Design review of the part built by this model. Coordinates are the model's own, in mm. A direction names the side the tool comes from. Give positions to 0.01 mm unless a question says otherwise; leave off trailing zeros. Write each loop counter-clockwise with the first axis right and the second up, starting at its lowest first coordinate (ties: lowest second). Pieces come first, ordered by that corner, then holes. Notation, with made-up numbers: (17.25, 44) -> (32.25, 44) arc R19 cw to (32.25, 58) -> close; hole circle Ø2 at (14.25, -36.75). An arc over 180 degrees is marked (long way). Answer as a JSON object with one key per item and string values.
Autodesk Inventor part; units mm, degrees
ref_plane "YZ Plane" through (0, 0, 0) normal (1, 0, 0) x (0, 1, 0)
ref_plane "XZ Plane" through (0, 0, 0) normal (0, 1, 0) x (-1, 0, 0)
ref_plane "XY Plane" through (0, 0, 0) normal (0, 0, 1) x (1, 0, 0)
sketch "Sketch1" plane through (0, 0, 0) normal (0, 0, 1) x (1, 0, 0)
  circle A0 centre (0, 0) radius 5.05
  circle A1 centre (0, 0) radius 15 construction
  line L0 (0, 0) -> (0, 15)
  circle A2 centre (0, 15) radius 2.5
  line L1 (2.4636, 15.425) -> (4.9765, 0.8585)
  line L2 (-4.9765, 0.8585) -> (-2.4636, 15.425)
  line L3 (0, 0) -> (-12.9904, -7.5)
  circle A3 centre (-12.9904, -7.5) radius 2.5
  line L4 (-14.5902, -5.579) -> (-3.2317, 3.8805)
  line L5 (1.7448, -4.739) -> (-12.1266, -9.846)
  line L6 (0, 0) -> (12.9904, -7.5)
  circle A4 centre (12.9904, -7.5) radius 2.5
  line L7 (12.1266, -9.846) -> (-1.7448, -4.739)
  line L8 (3.2317, 3.8805) -> (14.5902, -5.579)
  circle A5 centre (0, 0) radius 7.5
  point P0 (0, -15)
  point P1 (12.9904, 7.5)
  point P2 (-12.9904, 7.5)
  point P3 (-4.0338, 6.3228)
  point P4 (-3.4588, -6.6548)
  point P5 (3.4588, -6.6548)
  point P6 (4.0338, 6.3228)
  point P7 (7.4926, 0.332)
  point P8 (4.6604, 2.6907)
  point P9 (-7.4926, 0.332)
  point P10 (-4.6604, 2.6907)
  point P11 (0, -5.3814)
  dimension "d0" = 10.1
  dimension "d1" = 30
  dimension "d2" = 5
  dimension "d5" = 360
  dimension "d7" = 15
extrude "Extrusion1" add sketch "Sketch1" along normal blind 10 contours A0 L1 L8 A5 L6 | A0 L8 L1 | L6 A5 L7 L5 A0 | A0 L0 A5 L1 L8 | L1 A5 L8 | L5 L7 A0 | A5 L8 A4 L6 | L6 A4 L7 A5 | A0 L4 L2 A5 L0 | A5 L0 A2 L1 | L7 L5 A5 L3 A0 | L7 A5 L5 | L3 A5 L4 L2 A0 | A4 | A0 L2 L4 | A5 L2 A2 L0 | A2 | L5 A3 L3 A5 | L3 A3 L4 A5 | L4 A5 L2 | A3
extrude "Extrusion2" add sketch "Sketch1" along normal blind 2 contours A0 L6 L0 | A0 L3 L6 | L3 A0 L0
properties part number "Turret_Holder"
(1) For line 1 along X through (y, z) = (-2, 6); line 2 along X through (y, z) = (4.5, 5.5); line 3 along Z through (x, y) = (2, -3.75), list the stretches that pass through material, from the lowest coordinate up.
Here are the results:
{"line 1": "x = -10.29 to -4.64, 4.64 to 10.29", "line 2": "x = -6 to -2.29, 2.29 to 6", "line 3": "z = 0 to 2"}
(2) We need section C-C, the plane z = 1. State the section outline as (x, y) points (3 decimals).
Here are the results:
{"outline": "(-14.59, -5.579) arc R2.5 ccw to (-12.127, -9.846) -> (-3.459, -6.655) arc R7.5 ccw to (3.459, -6.655) -> (12.127, -9.846) arc R2.5 ccw to (14.59, -5.579) -> (7.493, 0.332) arc R7.5 ccw to (4.034, 6.323) -> (2.464, 15.425) arc R2.5 ccw to (-2.464, 15.425) -> (-4.034, 6.323) arc R7.5 ccw to (-7.493, 0.332) -> close"}
(3) The part is to be moulded in two halves that separate along X. For faces 1 (the cylindrical face through (6.47, 3.79, 4.93)), 2 (the cylindrical face through (0.1, -7.5, 4.9)), 3 (the flat face through (-11.091, -2.665, 4.93)), 4 (the flat face through (0, 0, 2)), say which applies: +X half, -X half, draft (parallel to the pull), parting line (faces both ways), or undercut.
Here are the results:
{"face 1": "+X half", "face 2": "undercut", "face 3": "-X half", "face 4": "undercut"}
(4) For faces 5 (the flat face through (7.85, -8.27, 4.93)), 6 (the flat face through (10.99, -2.58, 4.93)), list the 3-axis set-ups (+Z, -Z, +X, -X, +Y, -Y) from which the entire face can be reached by the end or side of a thin tool; tool diameter is ignored.
Here are the results:
{"face 5": "+Z, -Z, -Y", "face 6": "+Z, -Z, +X, +Y"}
(5) We need section D-D, the plane x = 11.5. State the section outline as (y, z) points.
Here are the results:
{"outline": "(-9.62, 0) -> (-3.01, 0) -> (-3.01, 10) -> (-9.62, 10) -> close"}
(6) Clearance check with flat-ended pins moving along their axes: pin 1 (5 mm diameter, centred on x = 0, y = -1, fed in from +Z); pin 2 (4 mm diameter, centred on x = 12, z = 4, fed in from +Y); pin 3 (3 mm diameter, centred on y = -1, z = 5.5, fed in from -X). State where each tip first meets the part, or that it passes through.
Here are the results:
{"pin 1": "stops at z = 2", "pin 2": "stops at y = -1.76", "pin 3": "stops at x = -10.89"}
(7) We need section B-B, the plane y = -0.5. State the section outline as (x, z) points.
Here are the results:
{"outline": "(-8.49, 0) -> (8.49, 0) -> (8.49, 10) -> (5.03, 10) -> (5.03, 2) -> (-5.03, 2) -> (-5.03, 10) -> (-8.49, 10) -> close"}
